Autodesk Inventor part; units mm, degrees
ref_plane "作業平面1" through (0, 0, 14) normal (0, 0, 1) x (-0.9659258, -0.258819, 0)
ref_plane "YZ Plane" through (0, 0, 0) normal (1, 0, 0) x (0, 1, 0)
ref_plane "XZ Plane" through (0, 0, 0) normal (0, 1, 0) x (-1, 0, 0)
ref_plane "作業平面1" through (0, 0, 14) normal (0, 0, 1) x (-0.9659258, -0.258819, 0)
sketch "スケッチ14" plane through (0, 0, 0) normal (0, 0, 1) x (1, 0, 0)
  circle A0 centre (0, 0) radius 25
  circle A1 centre (30, 0) radius 4.05
  line L0 (0, 25) -> (40, 25)
  line L1 (40, 25) -> (40, -25)
  line L2 (40, -25) -> (0, -25)
  line L3 (0, -25) -> (0, 25)
  line L4 (0, -25) -> (40, -10.4412)
  line L5 (0, 25) -> (40, 10.4412)
  line L6 (0.5157, 26.4168) -> (40.5157, 11.858)
  line L7 (0.5157, -26.4168) -> (40.5157, -11.858)
  circle A2 centre (0, 0) radius 6.5
  line L8 (40.5157, -11.858) -> (63.847, -3.366)
  line L9 (37.8689, 40.3876) -> (23.4147, 35.1267)
  line L10 (23.4147, 35.1267) -> (-16.5853, 20.5679)
  line L11 (-16.5853, 20.5679) -> (-32.0428, 14.9418)
  line L12 (-32.0428, 14.9418) -> (-14.9418, -32.0428)
  line L13 (-14.9418, -32.0428) -> (0.5157, -26.4168)
  line L14 (40, 12.0456) -> (47.7428, -9.2275)
  line L15 (40, 12.0456) -> (30.6418, 37.7571)
  point P0 (8.5505, -23.4923)
  point P1 (40, -12.0456)
  point P2 (40, 12.0456)
  point P3 (8.5505, 23.4923)
  dimension "d111" = 50
  dimension "d112" = 8.1
  dimension "d113" = 30
  dimension "d114" = 40
  dimension "d115" = 50
  dimension "d116" = 25
  dimension "d119" = 25
  dimension "d126" = 20
  dimension "d127" = 20
  dimension "d144" = 13
  dimension "d201" = 90
  dimension "d202" = 90
extrude "押し出し9" add sketch "スケッチ14" along normal blind 5 contours A0 L4 L3 A2 L5 | A0 L5 L1 L4 | L5 A0 | A0 L6 L1 L5 | L4 L1 L7 A0 | A0 L4 | L3 A2 A0
sketch "スケッチ15" plane through (0, 0, 0) normal (0, 0, -1) x (-1, 0, 0)
  circle A0 centre (-30, 0) radius 4.05
  circle A1 centre (-30, 0) radius 6.6
  line L0 (-24.4, 3.4928) -> (-24.4, -3.4928)
  arc A2 (-24.4, 1.4928) -> (-24.4, 3.4928) centre (-24.4, 2.4928) ccw
  arc A3 (-24.4, -3.4928) -> (-24.4, -1.4928) centre (-24.4, -2.4928) ccw
  point P0 (0, 0)
  dimension "d122" = 13.2
  dimension "d203" = 5.6
  dimension "d206" = 0
  dimension "d207" = 0
  dimension "d208" = 1
  dimension "d209" = 1
extrude "押し出し10" cut sketch "スケッチ15" against normal blind 2 contours L0 A1
sketch "スケッチ16" plane through (0, 0, 5) normal (0, 0, 1) x (1, 0, 0)
  circle A0 centre (30, 0) radius 4.05
  circle A1 centre (30, 0) radius 17
  arc A2 (8.5505, 23.4923) -> (8.5505, -23.4923) centre (0, 0) ccw
  circle A3 centre (0, 0) radius 25
  line L0 (40, -12.0456) -> (40, 12.0456)
  line L1 (40, 12.0456) -> (-0.2187, 26.6841)
  line L2 (40, -12.0456) -> (-2.6962, -27.5858)
  circle A4 centre (0, 0) radius 17.5
  line L3 (8.5505, 23.4923) -> (5.9854, 16.4446)
  line L4 (-17.5, 0) -> (-25, 0)
  line L5 (-2.7839, 19.6364) -> (32.5, 6.7941)
  line L6 (32.5, 6.7941) -> (32.5, -6.7941)
  line L7 (32.5, -6.7941) -> (-5.2613, -20.5381)
  line L8 (17.9474, 20.0721) -> (15.3823, 13.0244)
  line L9 (-17.5, 0) -> (0, 0)
  line L10 (-13.6656, -12.9367) -> (-0.4151, -19.1155)
  line L11 (-7.0404, -16.0261) -> (-11.4484, -25.4792)
  line L12 (17.2336, 18.1109) -> (11.4362, 13.2463)
  line L13 (18.0185, 5.7516) -> (7.3857, 18.4233)
  line L14 (0, 25) -> (0, 10.5586)
  line L15 (17.2336, 18.1109) -> (19.0798, 19.66)
  point P0 (0, -25)
  point P1 (-11.8057, -12.918)
  point P2 (-10.2087, -22.8207)
  point P3 (-7.3958, -15.8604)
  dimension "d125" = 34
  dimension "d128" = 7.5
  dimension "d164" = 7.5
  dimension "d165" = 10
  dimension "d186" = 90
  dimension "d187" = 65
  dimension "d196" = 30
extrude "押し出し11" add sketch "スケッチ16" along normal blind 12 contours L12 L5 L3 A3 | A3 L1 L8 | L8 L1 L15 | L3 L5 L14 A2 | L12 L13 L5 | A2 L4 A4 L10 L11 | L14 A4 L4 A2 | L5 L13 L12 A4 | A4 L14 L5
sketch "スケッチ17" plane through (0, 0, 5) normal (0, 0, 1) x (1, 0, 0)
  circle A0 centre (30, 0) radius 4.05
  line L0 (0, 0) -> (30, 0)
  circle A1 centre (0, 0) radius 12.5
  line L1 (0, 0) -> (12.4415, 7.1831)
  point P0 (10.8253, 6.25)
  point P1 (0, 12.5)
  point P2 (-10.8253, 6.25)
  point P3 (-10.8253, -6.25)
  point P4 (0, -12.5)
  point P5 (10.8253, -6.25)
  dimension "d131" = 25
  dimension "d132" = 30
  dimension "d135" = 360
hole "穴5" at (10.8253, 6.25, 5) at (0, 12.5, 5) at (-10.8253, 6.25, 5) at (-10.8253, -6.25, 5) at (0, -12.5, 5) at (10.8253, -6.25, 5) direction (0, 0, -1) diameter 3.2 end through all
sketch "スケッチ18" plane through (0, 0, 5) normal (0, 0, 1) x (1, 0, 0)
  circle A0 centre (30, 0) radius 4.05
  line L0 (0, 0) -> (30, 0)
  circle A1 centre (0, 0) radius 10.2
  point P0 (10.2, 0)
  point P1 (-5.1, 8.8335)
  point P2 (-5.1, -8.8335)
  dimension "d145" = 20.4
  dimension "d148" = 360
hole "穴6" at (10.2, 0, 5) at (-5.1, 8.8335, 5) at (-5.1, -8.8335, 5) direction (0, 0, -1) diameter 4.2 end through all
sketch "スケッチ19" plane through (0, 0, 5) normal (0, 0, 1) x (1, 0, 0)
  circle A0 centre (0, 12.5) radius 1.6
  circle A1 centre (0, 0) radius 12.5
  circle A2 centre (0, 12.5) radius 3
  circle A3 centre (-10.8253, 6.25) radius 3
  circle A4 centre (-10.8253, -6.25) radius 3
  circle A5 centre (0, -12.5) radius 3
  circle A6 centre (10.8253, -6.25) radius 3
  circle A7 centre (10.8253, 6.25) radius 3
  dimension "d157" = 6
  dimension "d160" = 360
extrude "押し出し12" cut sketch "スケッチ19" against normal blind 3 contours A0 A1 | A0 A1 A2 | A1 A0 | A0 A1 A2 | A3 A1 | A1 A3 | A7 A1 | A1 A7 | A4 A1 | A1 A4 | A6 A1 | A1 A6 | A5 A1 | A1 A5
sketch "スケッチ20" plane through (0, 0, 17) normal (0, 0, 1) x (1, 0, 0)
  line L0 (19.0798, 19.66) -> (8.5505, 23.4923)
  line L1 (17.9474, 20.0721) -> (15.3823, 13.0244)
  line L2 (15.3823, 13.0244) -> (5.9854, 16.4446)
  line L3 (5.9854, 16.4446) -> (8.5505, 23.4923)
  line L4 (0, 0) -> (0, 30.7788)
  circle A0 centre (0, 0) radius 21.25
  circle A1 centre (0, 0) radius 25
  point P0 (11.9664, 18.2584)
  point P1 (0, 21.25)
  point P2 (-10.625, 18.403)
  point P3 (-18.403, 10.625)
  point P4 (-21.25, 0)
  point P5 (-18.403, -10.625)
  point P6 (-10.625, -18.403)
  point P7 (0, -21.25)
  point P8 (10.625, -18.403)
  point P9 (18.403, -10.625)
  point P10 (21.25, 0)
  point P11 (18.403, 10.625)
  point P12 (10.625, 18.403)
  dimension "d167" = 7.5
  dimension "d168" = 5
  dimension "d169" = 3.75
  dimension "d170" = 3.75
  dimension "d171" = 50
  dimension "d174" = 360
hole "穴7" at (10.625, 18.403, 17) at (0, 21.25, 17) at (-10.625, 18.403, 17) at (-18.403, 10.625, 17) direction (0, 0, -1) diameter 2.459 depth 10
fillet "フィレット9" radius 17 2 edges at (40, 12.0456, 2.5) (40, -12.0456, 2.5)
sketch "スケッチ21" plane through (0, 0, 17) normal (0, 0, 1) x (1, 0, 0)
  circle A0 centre (-18.403, 10.625) radius 1.2295
  circle A1 centre (0, 0) radius 21.25
  line L0 (0, 0) -> (-31.1052, 0)
  point P0 (-21.25, 0)
  point P1 (-18.403, -10.625)
hole "穴8" at (-21.25, 0, 17) at (-18.403, -10.625, 17) direction (0, 0, -1) diameter 2.459 depth 10
fillet "フィレット12" radius 3.75 4 edges at (-7.0404, -16.0261, 11) (-10.2087, -22.8207, 11) (19.0798, 19.66, 11) (11.4362, 13.2463, 11)
mirror "ミラー1" about plane through (0, 0, 0) normal (0, 0, 1)
sketch "スケッチ22" plane through (0, 0, 17) normal (0, 0, 1) x (1, 0, 0)
  line L0 (-52.2093, 35.4502) -> (60.0334, 35.4502)
  line L1 (60.0334, 35.4502) -> (60.0334, -31.2)
  line L2 (60.0334, -31.2) -> (-52.2093, -31.2)
  line L3 (-52.2093, -31.2) -> (-52.2093, 35.4502)
  point P0 (0, 0)
extrude "押し出し13" cut sketch "スケッチ22" against normal blind 17
sketch "スケッチ23" plane through (0, 0, 0) normal (0, 0, 1) x (1, 0, 0)
  line L0 (24.4, 3.4928) -> (24.4, -3.4928)
  arc A0 (24.4, 3.4928) -> (24.4, 1.4928) centre (24.4, 2.4928) ccw
  arc A1 (24.4, -1.4928) -> (24.4, -3.4928) centre (24.4, -2.4928) ccw
  point P0 (0, 0)
  dimension "d210" = 0
  dimension "d211" = 1
  dimension "d212" = 0
  dimension "d213" = 1
extrude "押し出し14" cut sketch "スケッチ23" against normal blind 2
properties part number "RP_Thigh-Base_MIR" material "アルミニウム 6061"
Verification items for the finished model (mm, model axes). A direction names the side the tool comes from. Coordinates: 2 decimals unless noted, no trailing zeros. Order: outer loops, then holes, each group sorted by start corner. A loop starts at its lowest first (then second) coordinate and runs counter-clockwise, first axis right, second up.
Item 1: Section check A-A, the plane x = 0. Give the number of separate pieces and of enclosed holes in the cut face, then the cut area to 3 significant figures.
Filled in:
separate pieces: 4
enclosed holes: 0
area: 202 mm2
Item 2: Access from +Z, -Z, +X, -X, +Y, -Y to the whole of each face (thin tool, end or side, straight path). Record for faces 4 (the face through (-18.874, -11.761, -11.93)), 5 (the face through (-8.29, -16.63, -10.92)), 6 (the face through (36.596, -0.239, -0.986)).
Filled in:
face 4: -Z
face 5: -Z, +X
face 6: +Z
Item 3: Section check C-C, the plane x = 30. Enter the section's corners in (y, z), then the cut area to 3 significant figures.
Filled in:
outline: (-15.63, -5) - (-4.05, -5) - (-4.05, -2) - (-6.6, -2) - (-6.6, 0) - (-15.63, 0) - close; (4.05, -5) - (15.63, -5) - (15.63, 0) - (6.6, 0) - (6.6, -2) - (4.05, -2) - close
area: 106 mm2
Item 4: Material ranges on L1, parallel to X at y = 0, z = -3.05; L2, parallel to Y at x = 0, z = -2.4; L3, parallel to X at y = 10, z = -4, recorded low to high.
Filled in:
L1: x = -25 to -6.5, 6.5 to 8.1, 12.3 to 25.95, 34.05 to 40
L2: y = -25 to -15.5, -9.5 to -6.5, 6.5 to 9.5, 15.5 to 25
L3: x = -22.91 to -6.85, -3.35 to -1.66, 1.66 to 36.85
Item 5: Section check D-D, the plane y = -18. Enter the section's corners in (x, z).
Filled in:
outline: (-17.35, -17) - (-8.18, -17) - (-8.18, -5) - (23.64, -5) - (23.64, 0) - (-17.35, 0) - close
Item 6: Release check for a two-part mould opening along Y. For faces 1 (the face through (11.506, 14.267, -10.916)), 2 (the face through (13.687, 5.349, -3.521)), 3 (the face through (7, 0, 0)) record: +Y half, -Y half, draft (parallel to the pull), parting line (faces both ways), or undercut.
Filled in:
face 1: -Y half
face 2: undercut
face 3: draft
Item 7: Depth check by flat-ended pin: pin 1 (3 mm diameter, centred on x = -17.5, z = -11.5, fed in from +Y); pin 2 (3 mm diameter, centred on y = -16, z = -3.5, fed in from +X); pin 3 (2 mm diameter, centred on x = 1, z = -12.5, fed in from -Y). Enter the tip coordinate at first touch or a pass-through.
Filled in:
pin 1: stops at y = 19.21
pin 2: stops at x = 32.1
pin 3: stops at y = 17.39
